Can you work these out from the drawing? Everything is in mm from the part's minimum corner. A direction names the side the tool comes from. Coordinates: 2 decimals unless noted, no trailing zeros. Order: outer loops, then holes, each group sorted by start corner. A loop starts at its lowest first (then second) coordinate and runs counter-clockwise, first axis right, second up. Notation, with made-up numbers: M 80.5,28.5 L 122.5,28.5 A20 cw 122.5,43.5 Z; hole C 81,13 d8. An arc over 180 degrees is marked long. Answer as a JSON object with one key per item and string values.
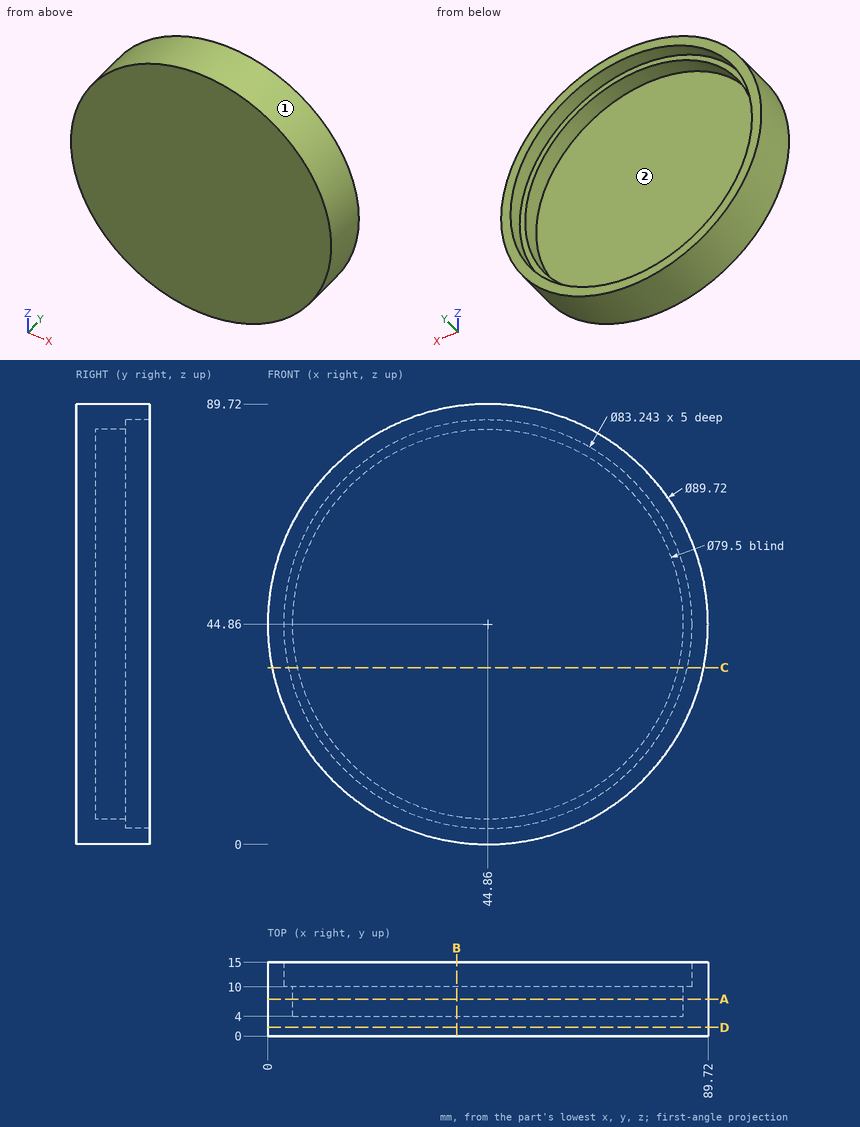
Item 1: I want a section at B-B, the plane x = 38.5. Write out the boundary of the cut face in (y, z).
Answers follow:
{"outline": "M 0,0.45 L 15,0.45 L 15,3.73 L 10,3.73 L 10,5.62 L 4,5.62 L 4,84.1 L 10,84.1 L 10,85.99 L 15,85.99 L 15,89.27 L 0,89.27 Z"}
Item 2: I want a section at A-A, the plane y = 7.5. Write out the boundary of the cut face in (x, z).
Answers follow:
{"outline": "C 44.86,44.86 d89.72; hole C 44.86,44.86 d79.5"}
Item 3: I'm going to push flat-ended pins straight in: pin 1 (6 mm diameter, centred on y = 8.5, z = 66, fed in from -X); pin 2 (3 mm diameter, centred on y = 13, z = 54.5, fed in from +X) (1 decimal); pin 3 (4 mm diameter, centred on x = 54, y = 10.5, fed in from -Z). Where does each tip first touch, or does it pass through?
Answers follow:
{"pin 1": "stops at x = 3.83", "pin 2": "stops at x = 89", "pin 3": "stops at z = 0.57"}
Item 4: Please list where these lines run through material, in increasing order: line 1 (Z direction, x = 44.86, y = 5.7); line 2 (Z direction, x = 44.86, y = 12.75); line 3 (Y direction, x = 55.5, z = 73).
Answers follow:
{"line 1": "z = 0 to 5.11, 84.61 to 89.72", "line 2": "z = 0 to 3.24, 86.48 to 89.72", "line 3": "y = 0 to 4"}
Item 5: I want a section at D-D, the plane y = 1.75. Write out the boundary of the cut face in (x, z), plus the area to 3 significant figures.
Answers follow:
{"outline": "C 44.86,44.86 d89.72", "area": "6,320 mm^2"}
Item 6: Which directions (+Z, -Z, +X, -X, +Y, -Y) give clear straight access to the entire face, cutting with the end or side of a thin tool? Please do the marked faces 1 and 2.
Answers follow:
{"face 1": "+Y, -Y", "face 2": "+Y"}
Item 7: I want a section at C-C, the plane z = 36. Write out the boundary of the cut face in (x, y).
Answers follow:
{"outline": "M 0.88,0 L 88.84,0 L 88.84,15 L 85.53,15 L 85.53,10 L 83.61,10 L 83.61,4 L 6.11,4 L 6.11,10 L 4.19,10 L 4.19,15 L 0.88,15 Z"}
